from build123d import *

# Parameters (mm, degrees)
SKETCH1_R           = 5
BOSS_EXTRUDE1_DEPTH = 5


with BuildPart() as part:
    # Sketch1 → Boss-Extrude1 (new, symmetric)
    with BuildSketch(Plane.XY):
        with BuildLine():
            Line((-83.738010361, 45.784514601), (-53.074190666, 45.784514601))
            Line((-53.074190666, 45.784514601), (-53.074190666, 15.784514601))
            Line((-53.074190666, 15.784514601), (-83.738010361, 15.784514601))
            ThreePointArc((-83.738010361, 15.784514601), (-98.738010361, 30.784514601), (-83.738010361, 45.784514601))
        make_face()
        with Locations((-83.738010361, 30.784514601)):
            Circle(SKETCH1_R, mode=Mode.SUBTRACT)
    extrude(amount=BOSS_EXTRUDE1_DEPTH, both=True)

    # Sketch2 → Revolve1 (revolve)
    with BuildSketch(Plane.XY.offset(5), mode=Mode.PRIVATE) as revolve1_sk:
        Polygon((-53.074190666, 45.784514601), (-53.074190666, 47.99778913), (-50.728429203, 47.99778913), (-50.728429203, 39.869151099), (162.360473408, 39.869151099), (162.360473408, 35.107489348), (-48.658763898, 35.107489348), (-48.658763898, 30.784514601), (-53.074190666, 30.784514601), align=None)
    revolve(revolve1_sk.sketch.rotate(Axis((-48.658763898, 30.784514601, 5), (-1, 0, 0)), 90), axis=Axis((-48.658763898, 30.784514601, 5), (-1, 0, 0)))


solid = part.part
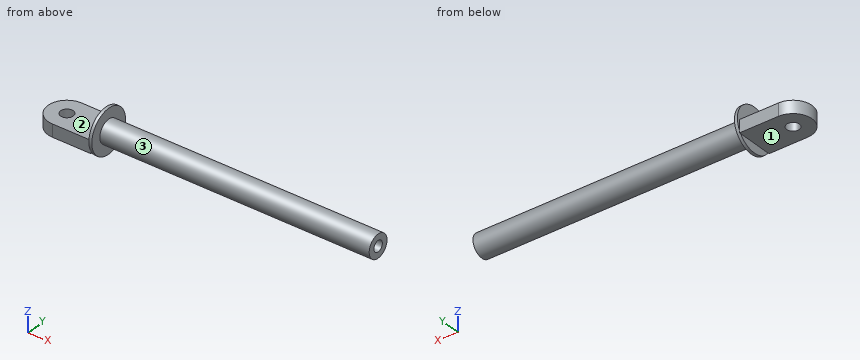
Part model, mm, in its own coordinate system. Face numbers are marked on the shaded views. A direction names the side the tool comes from. Round coordinates to 2 decimals unless told otherwise and drop trailing zeros. Write each loop counter-clockwise with the first axis right and the second up, starting at its lowest first coordinate (ties: lowest second). Pieces come first, ordered by that corner, then holes. Notation, with made-up numbers: M 73.5,-10.5 L 84.5,-10.5 A31 ccw 84.5,17.5 Z; hole C 83,-7.75 d2. An arc over 180 degrees is marked long. Return JSON: item names as keys, results as strings. Group by question number.
(1) Saw through at C-C on x = 80.5. Write the cut outline in (y, z), then the cut area to 3 significant figures.
(2) Saw through at B-B on z = -10. Write the cut outline in (x, y), then the cut area to 3 significant figures.
(3) Which spindle directions (+Z, -Z, +X, -X, +Y, -Y) get a long thin tool onto all of the face, cutting with end or side? Do the marked faces 1, 2 and 3. Say none if no direction does.
(4) Pin check, flat tips, straight feed: pin 1 Ø8 at (y, z) = (33.5, -7.5) entering from -X; pin 2 Ø3 at (x, z) = (57, -1.5) entering from -Y; pin 3 Ø10 at (x, z) = (40.5, 6) entering from -Y; pin 4 Ø2 at (x, y) = (58.5, 27) entering from -Z. Stop position of each tip, or through.
(5) Saw through at A-A on x = -62. Write the cut outline in (y, z).
(6) Drill centre lines: probe 1 along Y at (x, z) = (32, 5); probe 2 along Z at (x, y) = (42, 32); probe 3 along X at (y, z) = (28, 12). Where is each one in solid material? Low to high.
Returned:
{
 "1": {"outline": "C 30.78,5 d18.17; hole C 30.78,5 d8.65", "area": "201 mm²"},
 "2": {"outline": "M -53.07,22.34 L -50.73,22.34 L -50.73,39.23 L -53.07,39.23 Z", "area": "39.6 mm²"},
 "3": {"face 1": "-Z, -X, +Y, -Y", "face 2": "+Z, -X, +Y, -Y", "face 3": "+X"},
 "4": {"pin 1": "x = -98.74", "pin 2": "y = 23.2", "pin 3": "y = 21.7", "pin 4": "z = -3.65"},
 "5": {"outline": "M 15.78,-5 L 45.78,-5 L 45.78,5 L 15.78,5 Z"},
 "6": {"probe 1": "21.7 to 26.46, 35.11 to 39.87", "probe 2": "-4 to 0.85, 9.15 to 14", "probe 3": "-53.07 to 162.36"}
}
